Geometry: see drawing. Coordinates: mm, zero at the bounding-box minimum. A direction names the side the tool comes from. Give positions to 0.01 mm unless a question says otherwise; leave off trailing zeros. Loops run counter-clockwise (first coordinate to the right, second up) from the corner with the lowest first, then second, coordinate; pieces in that order, holes last. Notation, with made-up numbers: (15, -24) -> (28, -24) arc R21 cw to (28, 11) -> close; hole circle Ø10 at (25.5, -24.75). An arc over 180 degrees is marked (long way). Return JSON: item names as keys, results as strings. Group by question number.
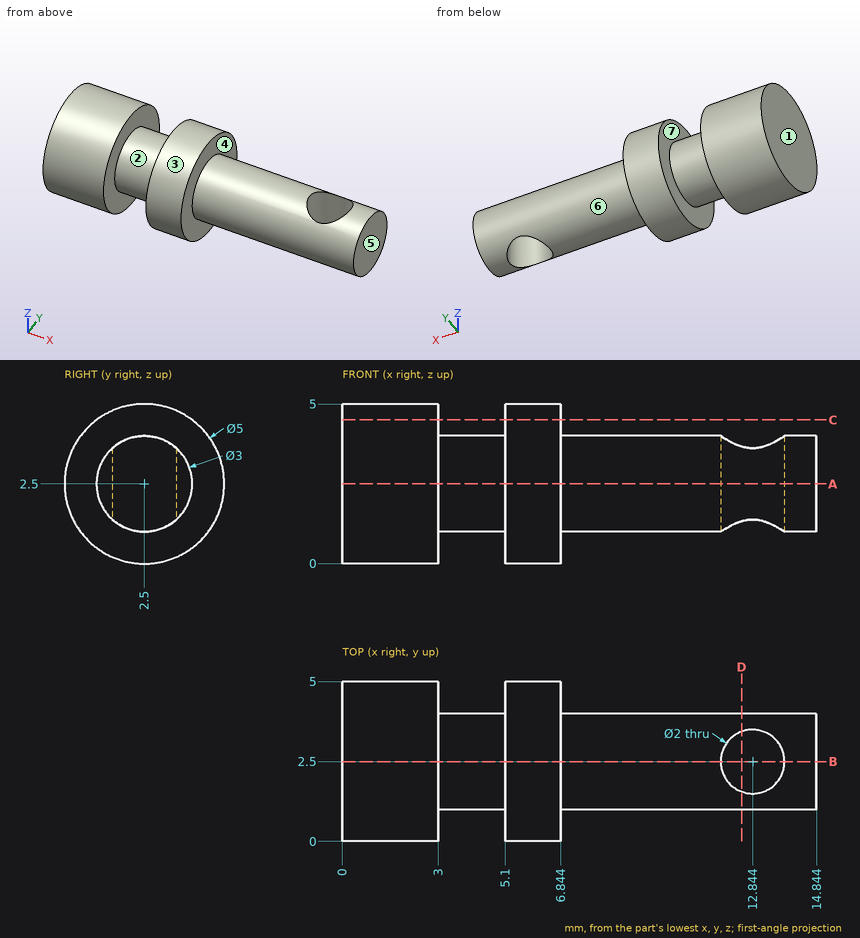
1) Cut plane B-B on y = 2.5. Return loops of the section in (x, z).
2) Mould query, pull axis X, two halves, no side actions, for the marked faces 1, 2, 3 and 4. Classes: released by +X, released by -X, zero draft, split by the parting line, or undercut.
3) Cut plane A-A on z = 2.5. Return loops of the section in (x, y), then the cut area to 3 significant figures.
4) Material intervals for line 1 (X direction, y = 2.5, z = 1.8); line 2 (X direction, y = 4.3, z = 4.2); line 3 (Z direction, x = 5.75, y = 1.9), sorted ascending.
5) Contact query for flat-ended pins moving along their axis: P1, Ø2, axis at x = 9.5, y = 0.5, coming from the -Z side; P2, Ø3, axis at x = 12.84, y = 2.5, coming from the +Z side. Output: stop coordinate, or through.
6) Cut plane D-D on x = 12.5. Return loops of the section in (y, z), then the cut area to 3 significant figures.
7) Reachability of the marked faces 5, 6 and 7 from +Z, -Z, +X, -X, +Y, -Y: full face, straight path, thin tool, end or side. Return the list, or none.
8) Cut plane C-C on z = 4.5. Return loops of the section in (x, y), then the cut area to 3 significant figures.
Calculated:
{
 "1": {"outline": "(0, 0) -> (3, 0) -> (3, 1) -> (5.1, 1) -> (5.1, 0) -> (6.84, 0) -> (6.84, 1) -> (11.84, 1) -> (11.84, 4) -> (6.84, 4) -> (6.84, 5) -> (5.1, 5) -> (5.1, 4) -> (3, 4) -> (3, 5) -> (0, 5) -> close; (13.84, 1) -> (14.84, 1) -> (14.84, 4) -> (13.84, 4) -> close"},
 "2": {"face 1": "released by -X", "face 2": "undercut", "face 3": "zero draft", "face 4": "released by +X"},
 "3": {"outline": "(0, 0) -> (3, 0) -> (3, 1) -> (5.1, 1) -> (5.1, 0) -> (6.84, 0) -> (6.84, 1) -> (14.84, 1) -> (14.84, 4) -> (6.84, 4) -> (6.84, 5) -> (5.1, 5) -> (5.1, 4) -> (3, 4) -> (3, 5) -> (0, 5) -> close; hole circle Ø2 at (12.84, 2.5)", "area": "50.9 mm2"},
 "4": {"line 1": "0 to 11.84, 13.84 to 14.84", "line 2": "0 to 3, 5.1 to 6.84", "line 3": "0.07 to 4.93"},
 "5": {"P1": "z = 1.38", "P2": "z = 4"},
 "6": {"outline": "(1.56, 1.33) -> (1.56, 3.67) arc R1.5 ccw to start; (3.44, 1.33) arc R1.5 ccw to (3.44, 3.67) -> close", "area": "1.83 mm2"},
 "7": {"face 5": "+Z, -Z, +X, +Y, -Y", "face 6": "+X", "face 7": "none"},
 "8": {"outline": "(0, 1) -> (3, 1) -> (3, 4) -> (0, 4) -> close; (5.1, 1) -> (6.84, 1) -> (6.84, 4) -> (5.1, 4) -> close", "area": "14.2 mm2"}
}
